Work out the finished part from the listing and answer in its coordinate system (mm). A direction names the side the tool comes from. Round coordinates to 2 decimals unless told otherwise and drop trailing zeros. Order: outer loops, then holes, each group sorted by start corner. A loop starts at its lowest first (then second) coordinate and runs counter-clockwise, first axis right, second up. Notation, with made-up numbers: (11, 76.5) - (68, 76.5) arc R13 cw to (68, 101.5) - close; hole circle Ø11 at (-13, -3). An arc over 180 degrees is marked (long way). Put each result on its own line as item: value.
```python
from build123d import *

# Parameters (mm, degrees)
SKETCH_1_W      = 30
SKETCH_1_H      = 20
SKETCH_1_R      = 2.15
SKETCH_1_W_2    = 8.956326716
SKETCH_1_H_2    = 15
EXTRUDE_1_DEPTH = 10
FILLET_1_R      = 1
FILLET_2_R      = 2


with BuildPart() as part:
    # 草图1 → 凸台-拉伸1 (new body)
    with BuildSketch(Plane.XY):
        Rectangle(SKETCH_1_W, SKETCH_1_H)
        with Locations((-10, 0)):
            Circle(SKETCH_1_R, mode=Mode.SUBTRACT)
        with Locations((10, 0)):
            Circle(SKETCH_1_R, mode=Mode.SUBTRACT)
        Rectangle(SKETCH_1_W_2, SKETCH_1_H_2, mode=Mode.SUBTRACT)
    extrude(amount=EXTRUDE_1_DEPTH)

    # 圆角1
    fillet_1_edges = [part.edges().sort_by_distance(p)[0] for p in [
        (4.478163358, -7.5, 5),
        (4.478163358, 7.5, 5),
        (-4.478163358, 7.5, 5),
        (-4.478163358, -7.5, 5),
    ]]
    fillet(fillet_1_edges, radius=FILLET_1_R)

    # 圆角2
    fillet_2_edges = [part.edges().sort_by_distance(p)[0] for p in [
        (15, -10, 5),
        (-15, -10, 5),
        (-15, 10, 5),
        (15, 10, 5),
    ]]
    fillet(fillet_2_edges, radius=FILLET_2_R)


solid = part.part
```
1) For faces 1 (the cylindrical face through (-14.43, -9.4, 5.07)), 2 (the flat face through (4.478, 0, 5)), determine the directions among +Z, -Z, +X, -X, +Y, -Y from which every point of the face is accessible in a straight line to the end or side of a thin tool.
Findings below:
face 1: +Z, -Z, -X, -Y
face 2: +Z, -Z
2) A cutting plane is placed at B-B on y = 0. Write down the section's boundary in (x, z), then the cut area to 3 significant figures.
Findings below:
outline: (-15, 0) - (-12.15, 0) - (-12.15, 10) - (-15, 10) - close; (-7.85, 0) - (-4.48, 0) - (-4.48, 10) - (-7.85, 10) - close; (4.48, 0) - (7.85, 0) - (7.85, 10) - (4.48, 10) - close; (12.15, 0) - (15, 0) - (15, 10) - (12.15, 10) - close
area: 124 mm2
3) For a pull along X with two mould halves and no side action, classify faces 3 (the flat face through (0, -10, 5)), 4 (the cylindrical face through (14.4, -9.43, 5.07)), 5 (the cylindrical face through (-4.18, -7.21, 5.07)), 6 (the flat face through (-15, 0, 5)) as pulls with the +X half, pulls with the -X half, needs draft (parallel to the pull), parting line crosses it, or undercut.
Findings below:
face 3: needs draft
face 4: pulls with the +X half
face 5: undercut
face 6: pulls with the -X half
4) Given pin 1 Ø1.5 at (x, y) = (2, 2.5) entering from +Z; pin 2 Ø4 at (x, y) = (-9, -7.5) entering from -Z, each flat-ended and moving along its own axis, determine where each tip first touches the part or whether it passes through.
Findings below:
pin 1: passes through
pin 2: stops at z = 0
5) A cutting plane is placed at A-A on x = -1.75. Write down the section's boundary in (y, z).
Findings below:
outline: (-10, 0) - (-7.5, 0) - (-7.5, 10) - (-10, 10) - close; (7.5, 0) - (10, 0) - (10, 10) - (7.5, 10) - close
6) A cutting plane is placed at C-C on y = 3.25. Write down the section's boundary in (x, z).
Findings below:
outline: (-15, 0) - (-4.48, 0) - (-4.48, 10) - (-15, 10) - close; (4.48, 0) - (15, 0) - (15, 10) - (4.48, 10) - close
7) Straight lines are drawn through the part: L1, parallel to Y at x = -3, z = 3; L2, parallel to X at y = 3, z = 2; L3, parallel to Y at x = 10, z = 7. For each, find the intervals that lie inside material, in ascending order. Write a range as from..to.
Findings below:
L1: y = -10..-7.5, 7.5..10
L2: x = -15..-4.48, 4.48..15
L3: y = -10..-2.15, 2.15..10
8) A cutting plane is placed at D-D on z = 3.75. Write down the section's boundary in (x, y), then the cut area to 3 significant figures.
Findings below:
outline: (-15, -8) arc R2 ccw to (-13, -10) - (13, -10) arc R2 ccw to (15, -8) - (15, 8) arc R2 ccw to (13, 10) - (-13, 10) arc R2 ccw to (-15, 8) - close; hole circle Ø4.3 at (-10, 0); hole (-4.48, -6.5) arc R1 ccw to (-3.48, -7.5) - (3.48, -7.5) arc R1 ccw to (4.48, -6.5) - (4.48, 6.5) arc R1 ccw to (3.48, 7.5) - (-3.48, 7.5) arc R1 ccw to (-4.48, 6.5) - close; hole circle Ø4.3 at (10, 0)
area: 434 mm2
